Here's how the part is built. I have some questions about the finished solid (model axes, mm). A direction names the side the tool comes from. Round coordinates to 2 decimals unless told otherwise and drop trailing zeros. Loops run counter-clockwise (first coordinate to the right, second up) from the corner with the lowest first, then second, coordinate; pieces in that order, holes last. Notation, with made-up numbers: M -21,30 L 35,30 A18 ccw 35,55 Z; hole C 49,-22 d3. An arc over 180 degrees is marked long. Use a Markdown table: item, result.
```python
from build123d import *

# Parameters (mm, degrees)
F0_W     = 700
F0_H     = 750
F0_W_2   = 640
F0_H_2   = 690
F1_DEPTH = 30
F2_W     = 30
F2_H     = 30
F3_DEPTH = 500
F6_DEPTH = 1000


with BuildPart() as f1:
    # F0 (on Right) → F1 (new body)
    with BuildSketch(Plane.YZ):
        with Locations((-143.150666, -375)):
            Rectangle(F0_W, F0_H)
        with Locations((-143.150666, -375)):
            Rectangle(F0_W_2, F0_H_2, mode=Mode.SUBTRACT)
    extrude(amount=F1_DEPTH)

    # F2 (on face) → F3 (join)
    with BuildSketch(Plane(origin=(0, 0, 0), x_dir=(0, -1, 0), z_dir=(-1, 0, 0))):
        with Locations((-6.849334, -15)):
            Rectangle(F2_W, F2_H)
    extrude(amount=F3_DEPTH)

    # F4: F1 across face


with BuildPart() as f1_1:
    add(f1.part)
    add(f1.part.mirror(Plane(origin=(-500, 6.849334, -15), x_dir=(0, -1, 0), z_dir=(-1, 0, 0))))

    # F5 (on face) → F6 (join, through all)
    with BuildSketch(Plane(origin=(0, 0, 0), x_dir=(0, -1, 0), z_dir=(-1, 0, 0))):
        Polygon((128.150666, -750), (143.150666, -750), (158.150666, -750), (158.150666, -720), (128.150666, -720), align=None)
    extrude(amount=F6_DEPTH)


solid = f1_1.part
```
Q1. Imagine slicing it at A-A, the plane x = -43. Please give me the cut outline in (y, z), then the cut area to 3 significant figures.
Return value:
| item | result |
|---|---|
| outline | M -158.15,-750 L -128.15,-750 L -128.15,-720 L -158.15,-720 Z; M -8.15,-30 L 21.85,-30 L 21.85,0 L -8.15,0 Z |
| area | 1,800 mm^2 |
Q2. For faces 1 (the flat face through (-493, -158.151, -735)), 2 (the flat face through (-498, -145, -750)), 3 (the flat face through (-1015, 176.849, -380)), 4 (the flat face through (-493, -128.151, -735)), which set-ups out of +Z, -Z, +X, -X, +Y, -Y let a thin tool reach every point of the face, with its end or its side?
Return value:
| item | result |
|---|---|
| face 1 | +Z, -Z, -Y |
| face 2 | -Z, +X, -X, +Y, -Y |
| face 3 | +X, -X |
| face 4 | +Z, -Z, +Y |
Q3. I need wall thicknesses on line 1 (X direction, y = -465, z = -676); line 2 (Z direction, x = -228, y = -129). Which ranges of each line are inside material? Lowest first, please. Write a range as from..to.
Return value:
| item | result |
|---|---|
| line 1 | x = -1030..-1000, 0..30 |
| line 2 | z = -750..-720 |
Q4. Imagine slicing it at C-C, the plane z = -376.5. Please give me the cut outline in (x, y), then the cut area to 3 significant figures.
Return value:
| item | result |
|---|---|
| outline | M -1030,-493.15 L -1000,-493.15 L -1000,-463.15 L -1030,-463.15 Z; M -1030,176.85 L -1000,176.85 L -1000,206.85 L -1030,206.85 Z; M 0,-493.15 L 30,-493.15 L 30,-463.15 L 0,-463.15 Z; M 0,176.85 L 30,176.85 L 30,206.85 L 0,206.85 Z |
| area | 3,600 mm^2 |
Q5. We'd pull the mould along Y, two halves only. Please class faces 5 (the flat face through (-458, -2, -30)), 6 (the flat face through (-507, 21.849, -15)), 7 (the flat face through (-1030, -482, -373)): pulls with the +Y half, pulls with the -Y half, needs draft (parallel to the pull), parting line crosses it, or undercut.
Return value:
| item | result |
|---|---|
| face 5 | undercut |
| face 6 | pulls with the +Y half |
| face 7 | needs draft |
Q6. Imagine slicing it at B-B, the plane y = -359.5. Please give me the cut outline in (x, z).
Return value:
| item | result |
|---|---|
| outline | M -1030,-750 L -1000,-750 L -1000,-720 L -1030,-720 Z; M -1030,-30 L -1000,-30 L -1000,0 L -1030,0 Z; M 0,-750 L 30,-750 L 30,-720 L 0,-720 Z; M 0,-30 L 30,-30 L 30,0 L 0,0 Z |
Q7. Will these pins go through, and if not, where does the flat tip stop? P1, Ø15, axis at x = -725, z = -18.5, coming from the +Y side; P2, Ø24, axis at x = -540, z = -735.5, coming from the -Y side; P3, Ø9, axis at x = -530, z = -8, coming from the -Y side.
Return value:
| item | result |
|---|---|
| P1 | stops at y = 21.85 |
| P2 | stops at y = -158.15 |
| P3 | stops at y = -8.15 |
